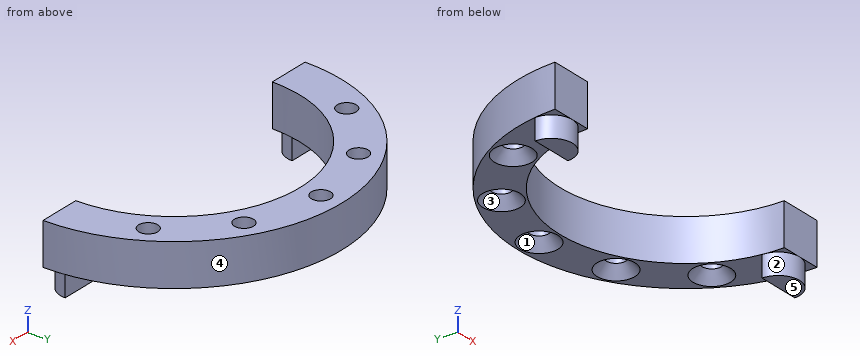
```python
from build123d import *

# Parameters (mm, degrees)
F1_DEPTH       = 12.7
F3_DEPTH       = 6.35
F5_D           = 5.7912
F5_CSINK_D     = 11.43
F5_CSINK_ANGLE = 82


with BuildPart() as f1:
    # F0 (on Top) → F1 (new body)
    with BuildSketch(Plane.XY):
        with BuildLine():
            ThreePointArc((50.8, 0), (0, 50.8), (-50.8, 0))
            Line((-50.8, 0), (-38.1, 0))
            ThreePointArc((-38.1, 0), (0, 38.1), (38.1, 0))
            Line((38.1, 0), (50.8, 0))
        make_face()
    extrude(amount=F1_DEPTH)

    # F2 (on Top) → F3 (join)
    with BuildSketch(Plane.XY):
        with BuildLine():
            Line((43.9940905122, 6.35), (37.6440905122, 6.35))
            ThreePointArc((37.6440905122, 6.35), (43.9940905122, 0), (50.3440905122, 6.35))
            Line((50.3440905122, 6.35), (43.9940905122, 6.35))
        make_face()
        with BuildLine():
            ThreePointArc((-50.3440905122, 6.35), (-43.9940905122, 0), (-37.6440905122, 6.35))
            Line((-37.6440905122, 6.35), (-43.9940905122, 6.35))
            Line((-43.9940905122, 6.35), (-50.3440905122, 6.35))
        make_face()
    extrude(amount=-F3_DEPTH)

    # F5 (through all)
    with Locations(Plane(origin=(0, 0, 0), x_dir=(1, 0, 0), z_dir=(0, 0, -1))):
        with Locations((-38.4948291982, -22.225), (-22.225, -38.4948291982), (0, -44.45), (22.225, -38.4948291982), (38.4948291982, -22.225)):
            CounterSinkHole(F5_D / 2, F5_CSINK_D / 2, counter_sink_angle=F5_CSINK_ANGLE)


solid = f1.part
```
The listing builds one solid part. Answer for the finished solid, in the listing's coordinates (mm). Face numbers are marked on the shaded views. A direction names the side the tool comes from. Round coordinates to 2 decimals unless told otherwise and drop trailing zeros. Loops run counter-clockwise (first coordinate to the right, second up) from the corner with the lowest first, then second, coordinate; pieces in that order, holes last. Notation, with made-up numbers: (72, 59) - (124, 59) arc R19 cw to (124, 79) - close; hole circle Ø5 at (-5.75, -1.5). An arc over 180 degrees is marked (long way). Return JSON: item names as keys, results as strings. Group by question number.
1. The part is cut by section C-C on z = 11.25. Determine the outline of the cut face in (x, y) (3 decimals), then the cut area to 3 significant figures.
2. The mould has two halves that part along Y. Classify the marked faces 3, 4 and 5: pulls with the +Y half, pulls with the -Y half, needs draft (parallel to the pull), parting line crosses it, or undercut.
3. Which of the six approach directions +Z, -Z, +X, -X, +Y, -Y give full straight-line access (tool end or side, diameter ignored) to the marked faces 1 and 2?
4. The part is cut by section A-A on x = 0. Determine the outline of the cut face in (y, z) (3 decimals), then the cut area to 3 significant figures.
5. Consider probe 1 along X at (y, z) = (35, 0.75); probe 2 along Y at (x, z) = (0, 9); probe 3 along X at (y, z) = (17.5, 5.5). Determine where each line is inside the solid, lowest interval first.
6. The part is cut by section D-D on y = 31. Determine the outline of the cut face in (x, z).
7. Each of these flat-tipped pins is pushed along its axis until it touches: P1, Ø3, axis at x = 28.5, z = 3.5, coming from the -Y side; P2, Ø7.5, axis at x = 0, y = 44.45, coming from the -Z side; P3, Ø1, axis at x = -7.5, z = 0, coming from the -Y side. Where does it stop, or does it pass through?
8. The part is cut by section B-B on y = 11.5. Determine the outline of the cut face in (x, z), then the cut area to 3 significant figures.
Resolved:
{
 "1": {"outline": "(-50.8, 0) - (-38.1, 0) arc R38.1 cw to (38.1, 0) - (50.8, 0) arc R50.8 ccw to start; hole circle Ø5.791 at (-38.495, 22.225); hole circle Ø5.791 at (-22.225, 38.495); hole circle Ø5.791 at (0, 44.45); hole circle Ø5.791 at (22.225, 38.495); hole circle Ø5.791 at (38.495, 22.225)", "area": "1,640 mm²"},
 "2": {"face 3": "undercut", "face 4": "pulls with the +Y half", "face 5": "needs draft"},
 "3": {"face 1": "-Z", "face 2": "-Z, -Y"},
 "4": {"outline": "(38.1, 0) - (38.735, 0) - (41.554, 3.243) - (41.554, 12.7) - (38.1, 12.7) - close; (47.346, 3.243) - (50.165, 0) - (50.8, 0) - (50.8, 12.7) - (47.346, 12.7) - close", "area": "78.6 mm²"},
 "5": {"probe 1": "x = -36.82 to -25.89, -18.56 to -15.05, 15.05 to 18.56, 25.89 to 36.82", "probe 2": "y = 38.1 to 41.55, 47.35 to 50.8", "probe 3": "x = -47.69 to -33.84, 33.84 to 47.69"},
 "6": {"outline": "(-40.24, 0) - (-22.15, 0) - (-22.15, 12.7) - (-40.24, 12.7) - close; (22.15, 0) - (40.24, 0) - (40.24, 12.7) - (22.15, 12.7) - close"},
 "7": {"P1": "stops at y = 23.49", "P2": "stops at z = 2.26", "P3": "stops at y = 37.25"},
 "8": {"outline": "(-49.48, 0) - (-36.32, 0) - (-36.32, 12.7) - (-49.48, 12.7) - close; (36.32, 0) - (49.48, 0) - (49.48, 12.7) - (36.32, 12.7) - close", "area": "334 mm²"}
}
